Answer from the drawing. Dimensions are ordinates in mm from the lowest x, y and z of the part. Give positions to 0.01 mm unless a question says otherwise; leave off trailing zeros. Loops run counter-clockwise (first coordinate to the right, second up) from the corner with the lowest first, then second, coordinate; pieces in that order, holes last.
(1) Find section B-B, the plane x = 3.5. Write down the section's boundary in (y, z).
(2) This flat-tipped pin is pushed along its axis until it touches: P1, Ø2.5, axis at x = 3.5, y = 81.5, coming from the +Z side. Where does it stop, or does it pass through?
(3) Straight lines are drawn through the part: probe 1 along Y at (x, z) = (3.5, 1.15); probe 2 along X at (y, z) = (81.5, 1.55); probe 3 along Y at (x, z) = (53, 0.25). For each, find the intervals that lie inside material, in ascending order.
(4) Find section A-A, the plane y = 23.5. Write down the section's boundary in (x, z).
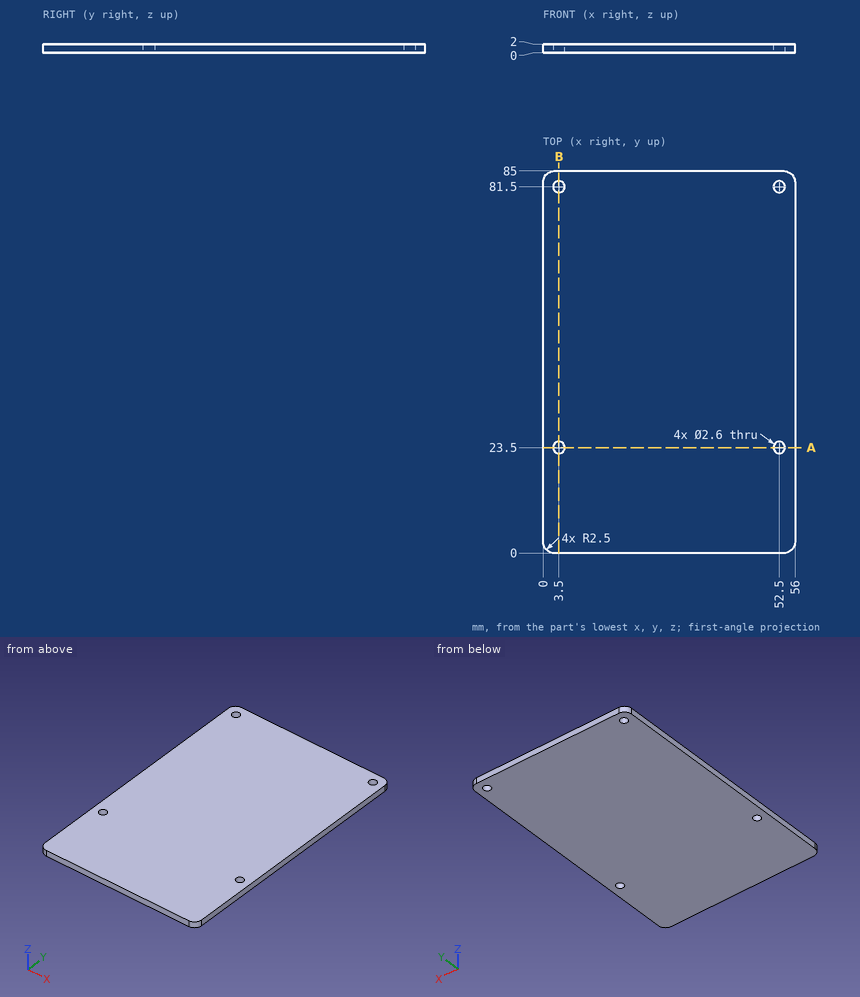
Entries:
1. outline: (0, 0) - (22.2, 0) - (22.2, 2) - (0, 2) - close; (24.8, 0) - (80.2, 0) - (80.2, 2) - (24.8, 2) - close; (82.8, 0) - (85, 0) - (85, 2) - (82.8, 2) - close
2. P1: passes through
3. probe 1: y = 0 to 22.2, 24.8 to 80.2, 82.8 to 85
3. probe 2: x = 0 to 2.2, 4.8 to 51.2, 53.8 to 56
3. probe 3: y = 0 to 22.3, 24.7 to 80.3, 82.7 to 85
4. outline: (0, 0) - (2.2, 0) - (2.2, 2) - (0, 2) - close; (4.8, 0) - (51.2, 0) - (51.2, 2) - (4.8, 2) - close; (53.8, 0) - (56, 0) - (56, 2) - (53.8, 2) - close
